from build123d import *

# Parameters (mm, degrees)
EXTRUDE_DEPTH                     = 6
EXTRUDE_ONTO_SKETCH039_ROLL_ANGLE = 90
SKETCH041_R                       = 1.7
POCKET009_DEPTH                   = 6
PAD006_DEPTH                      = 50
CHAMFER009_SIZE                   = 5
SKETCH043_W                       = 4
SKETCH043_H                       = 2
PAD007_DEPTH                      = 54
POCKET010_DEPTH                   = 50
POCKET011_DEPTH                   = 12
SKETCH047_W                       = 16.5
SKETCH047_H                       = 4.5
POCKET012_DEPTH                   = 50
SKETCH048_R                       = 1.65
POCKET013_DEPTH                   = 10
POCKET014_DEPTH                   = 16


with BuildPart() as part:
    # Sketch039 as drawn → Extrude (new)
    with BuildSketch(Plane.XY):
        Polygon((44.672363, 146.349121), (88.672363, 146.349121), (93.172363, 141.849121), (93.172363, 81.849121), (88.672363, 77.349121), (44.672363, 77.349121), (40.172363, 81.849121), (40.172363, 141.849121), align=None)
    extrude(amount=EXTRUDE_DEPTH)


with BuildPart() as part_1:
    # Extrude onto Sketch039 roll: moved
    add(part.part.rotate(Axis((0, 0, 0), (1, 0, 0)), EXTRUDE_ONTO_SKETCH039_ROLL_ANGLE))


with BuildPart() as part_2:
    # Extrude onto Sketch039 placement: moved
    add(part_1.part.moved(Location((-7, -30, 20))))

    # Sketch041 → Pocket009 (cut)
    with BuildSketch(Plane.XZ.offset(36)):
        with Locations((47.672363, 142.849121)):
            Circle(SKETCH041_R)
        with Locations((71.672363, 142.849121)):
            Circle(SKETCH041_R)
    extrude(amount=-POCKET009_DEPTH, mode=Mode.SUBTRACT)

    # Sketch042 → Pad006 (new body)
    with BuildSketch(Plane.XZ.offset(36)):
        Polygon((33.172363, 112.349121), (86.172363, 112.349121), (86.172363, 101.849121), (81.672363, 97.349121), (37.672363, 97.349121), (33.172363, 101.849121), align=None)
    extrude(amount=PAD006_DEPTH)

    # Chamfer009
    chamfer009_edges = [part_2.edges().sort_by_distance(p)[0] for p in [
        (86.172363, -86, 107.099121),
        (33.172363, -86, 107.099121),
    ]]
    chamfer(chamfer009_edges, length=CHAMFER009_SIZE)

    # Sketch043 → Pad007 (new body)
    with BuildSketch(Plane.XY.offset(166.349121)):
        with Locations((39.672363, -37)):
            Rectangle(SKETCH043_W, SKETCH043_H)
        with Locations((79.672363, -37)):
            Rectangle(SKETCH043_W, SKETCH043_H)
        with Locations((59.672363, -37)):
            Rectangle(SKETCH043_W, SKETCH043_H)
    extrude(amount=-PAD007_DEPTH)

    # Sketch044 → Pocket010 (cut)
    with BuildSketch(Plane.XZ.offset(86)):
        Polygon((38.172363, 97.349121), (41.233486, 100.410242), (78.111243, 100.410242), (81.172363, 97.349121), align=None)
    extrude(amount=-POCKET010_DEPTH, mode=Mode.SUBTRACT)

    # Sketch046 → Pocket011 (cut)
    with BuildSketch(Plane.XY.offset(112.349121)):
        Polygon((41.172363, -73.752892), (41.172363, -53.247108), (43.556055, -50.5), (75.788672, -50.5), (78.172363, -53.247108), (78.172363, -73.752892), (75.788672, -76.5), (43.556055, -76.5), align=None)
    extrude(amount=-POCKET011_DEPTH, mode=Mode.SUBTRACT)

    # Sketch047 → Pocket012 (cut)
    with BuildSketch(Plane.XZ.offset(86)):
        with Locations((59.672363, 110.099121)):
            Rectangle(SKETCH047_W, SKETCH047_H)
    extrude(amount=-POCKET012_DEPTH, mode=Mode.SUBTRACT)

    # Sketch048 → Pocket013 (cut)
    with BuildSketch(Plane.XY.offset(107.849121)):
        with Locations((59.672363, -80)):
            Circle(SKETCH048_R)
        with Locations((59.672363, -48)):
            Circle(SKETCH048_R)
    extrude(amount=-POCKET013_DEPTH, mode=Mode.SUBTRACT)

    # Sketch049 → Pocket014 (cut, symmetric)
    with BuildSketch(Plane(origin=(49.845623, -43.251529, 0), x_dir=(0.65538, 0.755299, 0), z_dir=(0.755299, -0.65538, 0))):
        with BuildLine():
            ThreePointArc((-15.415378, 112.349121), (-11.415378, 108.349121), (-7.415378, 112.349121))
            Line((-15.415378, 112.349121), (-7.415378, 112.349121))
        make_face()
    extrude(amount=POCKET014_DEPTH, both=True, mode=Mode.SUBTRACT)


solid = part_2.part
Verification items for the finished model (mm, model axes). A direction names the side the tool comes from. Give positions to 0.01 mm unless a question says otherwise; leave off trailing zeros. Order: outer loops, then holes, each group sorted by start corner. A loop starts at its lowest first (then second) coordinate and runs counter-clockwise, first axis right, second up. Notation, with made-up numbers: M 12.25,-1 L 54.25,-1 A32 cw 54.25,36 Z; hole C 36.25,8.5 d4. An arc over 180 degrees is marked long. Use one line per item in the form item = value. Start each with the question number.
Q1. Section check B-B (x = 53). Enter the section's corners in (y, z).
Q2. Access from +Z, -Z, +X, -X, +Y, -Y to the whole of each face (thin tool, end or side, straight path). Record for faces 4 (the flat face through (60, -38, 140)), 5 (the flat face through (78.172, -63, 106)), 6 (the flat face through (57.672, -37, 140)), 7 (the flat face through (35, -36, 140)).
Q3. Section check C-C (z = 138). Enter the section's corners in (x, y).
Q4. Go/stop test with flat-tipped pins: pin 1 Ø3.5 at (x, z) = (83.5, 152) entering from -Y; pin 2 Ø9 at (x, y) = (76, -54.5) entering from +Z; pin 3 Ø3 at (x, z) = (41.5, 139.5) entering from -Y. Record where each tip stops, or that it passes through.
Q5. Section check A-A (y = -80). Enter the section's corners in (x, z), then the cut area to 3 significant figures.
Q6. Mould release check, pull along X, two halves, no side actions. Record for faces 1 (the flat face through (84, -36, 140)), 2 (the flat face through (76.96, -51.85, 106.43)), 3 (the flat face through (83.71, -83.46, 104.95)): +X half, -X half, draft (parallel to the pull), parting line (faces both ways), or undercut.
Q7. Scan lines: line 1 along X through (y, z) = (-80, 106.5); line 2 along X through (y, z) = (-66, 108); line 3 along Y through (x, z) = (64, 132). Record each from-to range of solid material in increasing order. Write a range as [from, to].
Q8. Section check D-D (z = 111). Enter the section's corners in (x, y).
Evaluation:
q1.outline = M -86,100.41 L -76.5,100.41 L -76.5,107.85 L -86,107.85 Z; M -50.5,100.41 L -36,100.41 L -36,97.35 L -30,97.35 L -30,166.35 L -36,166.35 L -36,107.85 L -50.5,107.85 Z
q2.face_4 = +Z, +X, -X, -Y
q2.face_5 = +Z, -Z
q2.face_6 = +Z, -Y
q2.face_7 = +Z, -X, -Y
q3.outline = M 33.17,-36 L 37.67,-36 L 37.67,-38 L 41.67,-38 L 41.67,-36 L 57.67,-36 L 57.67,-38 L 61.67,-38 L 61.67,-36 L 77.67,-36 L 77.67,-38 L 81.67,-38 L 81.67,-36 L 86.17,-36 L 86.17,-30 L 33.17,-30 Z
q4.pin_1 = -36
q4.pin_2 = 112.35
q4.pin_3 = -38
q5.outline = M 33.17,101.85 L 37.67,97.35 L 38.17,97.35 L 41.23,100.41 L 58.02,100.41 L 58.02,107.85 L 51.42,107.85 L 51.42,112.35 L 33.17,112.35 Z; M 61.32,100.41 L 78.11,100.41 L 81.17,97.35 L 81.67,97.35 L 86.17,101.85 L 86.17,112.35 L 67.92,112.35 L 67.92,107.85 L 61.32,107.85 Z
q5.area = 554 mm2
q6.face_1 = draft
q6.face_2 = undercut
q6.face_3 = +X half
q7.line_1 = [33.17, 58.02], [61.32, 86.17]
q7.line_2 = [33.17, 41.17], [78.17, 86.17]
q7.line_3 = [-36, -30]
q8.outline = M 33.17,-81 L 38.17,-86 L 51.42,-86 L 51.42,-76.5 L 43.56,-76.5 L 41.17,-73.75 L 41.17,-55.82 L 33.17,-48.88 Z; M 33.17,-38.91 L 46.53,-50.5 L 51.42,-50.5 L 51.42,-36 L 67.92,-36 L 67.92,-50.5 L 75.79,-50.5 L 78.17,-53.25 L 78.17,-73.75 L 75.79,-76.5 L 67.92,-76.5 L 67.92,-86 L 81.17,-86 L 86.17,-81 L 86.17,-30 L 33.17,-30 Z
